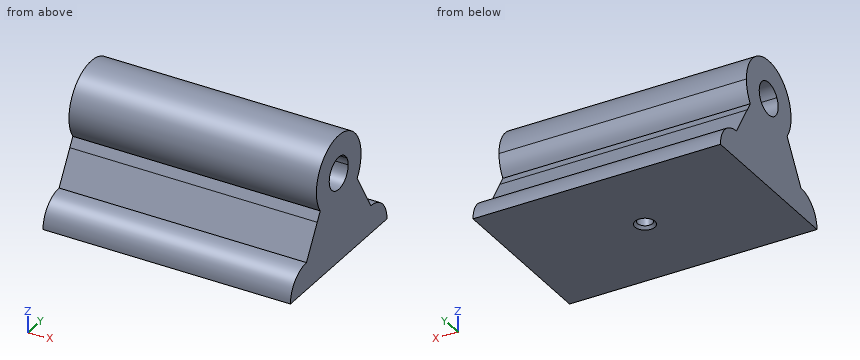
from build123d import *

# Parameters (mm, degrees)
F0_W           = 8.4991231561
F0_H           = 6.35
F1_DEPTH       = 57.15
F3_D           = 3.4544
F3_DEPTH       = 12.7
F3_CSINK_D     = 4.5974
F3_CSINK_ANGLE = 82
F3_TIP         = 1.0378064612


with BuildPart() as f1:
    # F0 (on Right) → F1 (new body)
    with BuildSketch(Plane.YZ):
        with BuildLine():
            Line((-8.4991231561, 2.5336752819), (-12.7344833851, 2.5336752819))
            ThreePointArc((-12.7344833851, 2.5336752819), (-17.2246114456, 0.6738033425), (-19.0844833851, -3.8163247181))
            Line((-19.0844833851, -3.8163247181), (-8.4991231561, -3.8163247181))
            Line((-8.4991231561, -3.8163247181), (-8.4991231561, 2.5336752819))
        make_face()
        with Locations((-4.249561578, -0.6413247181)):
            Rectangle(F0_W, F0_H)
        with Locations((4.249561578, -0.6413247181)):
            Rectangle(F0_W, F0_H)
        with BuildLine():
            ThreePointArc((19.0844833851, -3.8163247181), (17.2246114456, 0.6738033425), (12.7344833851, 2.5336752819))
            Line((12.7344833851, 2.5336752819), (8.4991231561, 2.5336752819))
            Line((8.4991231561, 2.5336752819), (8.4991231561, -3.8163247181))
            Line((8.4991231561, -3.8163247181), (19.0844833851, -3.8163247181))
        make_face()
        with BuildLine():
            ThreePointArc((8.4901041675, 9.7145254963), (0, 5.7086752819), (-8.4901041675, 9.7145254963))
            Line((-8.4901041675, 9.7145254963), (-12.7344833851, 2.5336752819))
            Line((-12.7344833851, 2.5336752819), (-8.4991231561, 2.5336752819))
            Line((-8.4991231561, 2.5336752819), (0, 2.5336752819))
            Line((0, 2.5336752819), (8.4991231561, 2.5336752819))
            Line((8.4991231561, 2.5336752819), (12.7344833851, 2.5336752819))
            Line((12.7344833851, 2.5336752819), (8.4901041675, 9.7145254963))
        make_face()
        with BuildLine():
            Line((-7.2959219906, 11.7349018344), (-8.4901041675, 9.7145254963))
            ThreePointArc((-8.4901041675, 9.7145254963), (0, 5.7086752819), (8.4901041675, 9.7145254963))
            Line((8.4901041675, 9.7145254963), (7.2959219906, 11.7349018344))
            ThreePointArc((7.2959219906, 11.7349018344), (0, 7.8786752819), (-7.2959219906, 11.7349018344))
        make_face()
        with BuildLine():
            ThreePointArc((8.83, 16.7086752819), (-2.6024900406, 25.1464442755), (-7.2959219906, 11.7349018344))
            Line((-7.2959219906, 11.7349018344), (-3.2282481135, 18.6167932336))
            ThreePointArc((-3.2282481135, 18.6167932336), (0, 20.4586752819), (3.2282481135, 18.6167932336))
            Line((3.2282481135, 18.6167932336), (7.2959219906, 11.7349018344))
            ThreePointArc((7.2959219906, 11.7349018344), (8.4377689935, 14.1061852413), (8.83, 16.7086752819))
        make_face()
        with BuildLine():
            Line((-3.2282481135, 18.6167932336), (-7.2959219906, 11.7349018344))
            ThreePointArc((-7.2959219906, 11.7349018344), (0, 7.8786752819), (7.2959219906, 11.7349018344))
            Line((7.2959219906, 11.7349018344), (3.2282481135, 18.6167932336))
            ThreePointArc((3.2282481135, 18.6167932336), (3.6172109716, 17.6977580829), (3.75, 16.7086752819))
            ThreePointArc((3.75, 16.7086752819), (-0.9890828009, 13.0914643104), (-3.2282481135, 18.6167932336))
        make_face()
    extrude(amount=-F1_DEPTH)

    # F3
    with Locations(Plane(origin=(0, 0, -3.8163247181), x_dir=(1, 0, 0), z_dir=(0, 0, -1))):
        with Locations((-28.575, 0)):
            CounterSinkHole(F3_D / 2, F3_CSINK_D / 2, depth=F3_DEPTH, counter_sink_angle=F3_CSINK_ANGLE)
            with Locations((0, 0, -(F3_DEPTH + F3_TIP / 2))):  # 118° drill point
                Cone(0, F3_D / 2, F3_TIP, mode=Mode.SUBTRACT)


solid = f1.part
Geometry check sheet. Reference: the model listing, model coordinates, mm. Give positions to 0.01 mm unless a question says otherwise; leave off trailing zeros. Loops run counter-clockwise (first coordinate to the right, second up) from the corner with the lowest first, then second, coordinate; pieces in that order, holes last. Notation, with made-up numbers: (69.5, 60.25) -> (87.5, 60.25) arc R21 ccw to (87.5, 70.25) -> close; hole circle Ø5 at (43, -19). An arc over 180 degrees is marked (long way). Answer in a Markdown table with one row per item. Add a question column.
1) Cross-section at D-D on z = 15.5. Record the boundary of the cut face in (x, y), and give its area (3 significant figures).
2) Material ranges on probe 1 along Y at (x, z) = (-19, 16.5); probe 2 along Z at (x, y) = (-33, 3); probe 3 along Z at (x, y) = (-53.5, 13), recorded low to high. Write a range as from..to.
3) Cross-section at C-C on z = 1.25. Record the boundary of the cut face in (x, y) (3 decimals).
4) Gauge pin test, flat ends, axial feed: P1, Ø4, axis at x = -21.5, z = 15, coming from the -Y side; P2, Ø1, axis at x = -23.5, z = 14, coming from the +Y side; P3, Ø1, axis at x = -40, y = -7, coming from the +Z side. Record the tip position at first contact, or that the pin passes through.
5) Cross-section at A-A on x = -17. Record the boundary of the cut face in (y, z), and give its area (3 significant figures).
6) Cross-section at B-B on z = 19.5. Record the boundary of the cut face in (x, y), and give its area (3 significant figures).
Outcome:
| question | item | result |
|---|---|---|
| 1 | outline | (-57.15, -8.75) -> (0, -8.75) -> (0, -3.55) -> (-57.15, -3.55) -> close; (-57.15, 3.55) -> (0, 3.55) -> (0, 8.75) -> (-57.15, 8.75) -> close |
| 1 | area | 594 mm^2 |
| 2 | probe 1 | y = -8.83..-3.74, 3.74..8.83 |
| 2 | probe 2 | z = -3.82..14.46, 18.96..25.01 |
| 2 | probe 3 | z = -3.82..2.53 |
| 3 | outline | (-57.15, -16.563) -> (0, -16.563) -> (0, 16.563) -> (-57.15, 16.563) -> close; hole circle Ø3.454 at (-28.575, 0) |
| 4 | P1 | stops at y = -8.83 |
| 4 | P2 | stops at y = 8.55 |
| 4 | P3 | stops at z = 22.69 |
| 5 | outline | (-19.08, -3.82) -> (19.08, -3.82) arc R6.35 ccw to (12.73, 2.53) -> (7.3, 11.73) arc R8.83 ccw (long way) to (-7.3, 11.73) -> (-12.73, 2.53) arc R6.35 ccw to start; hole circle Ø7.5 at (0, 16.71) |
| 5 | area | 571 mm^2 |
| 6 | outline | (-57.15, -8.38) -> (0, -8.38) -> (0, -2.5) -> (-57.15, -2.5) -> close; (-57.15, 2.5) -> (0, 2.5) -> (0, 8.38) -> (-57.15, 8.38) -> close |
| 6 | area | 671 mm^2 |
